Check sheet for the drawn part. Datum: minimum x, y, z corner. Units: mm. A direction names the side the tool comes from. Coordinates: 2 decimals unless noted, no trailing zeros. Loops run counter-clockwise (first coordinate to the right, second up) from the corner with the lowest first, then second, coordinate; pieces in that order, holes last. Notation, with made-up numbers: (32.5, -22.75) - (89.5, -22.75) arc R15 ccw to (89.5, -8.75) - close; hole circle Ø6 at (44.5, -25). An arc over 180 degrees is marked (long way). Answer as a JSON object with one key per item and string values. Group by question number.
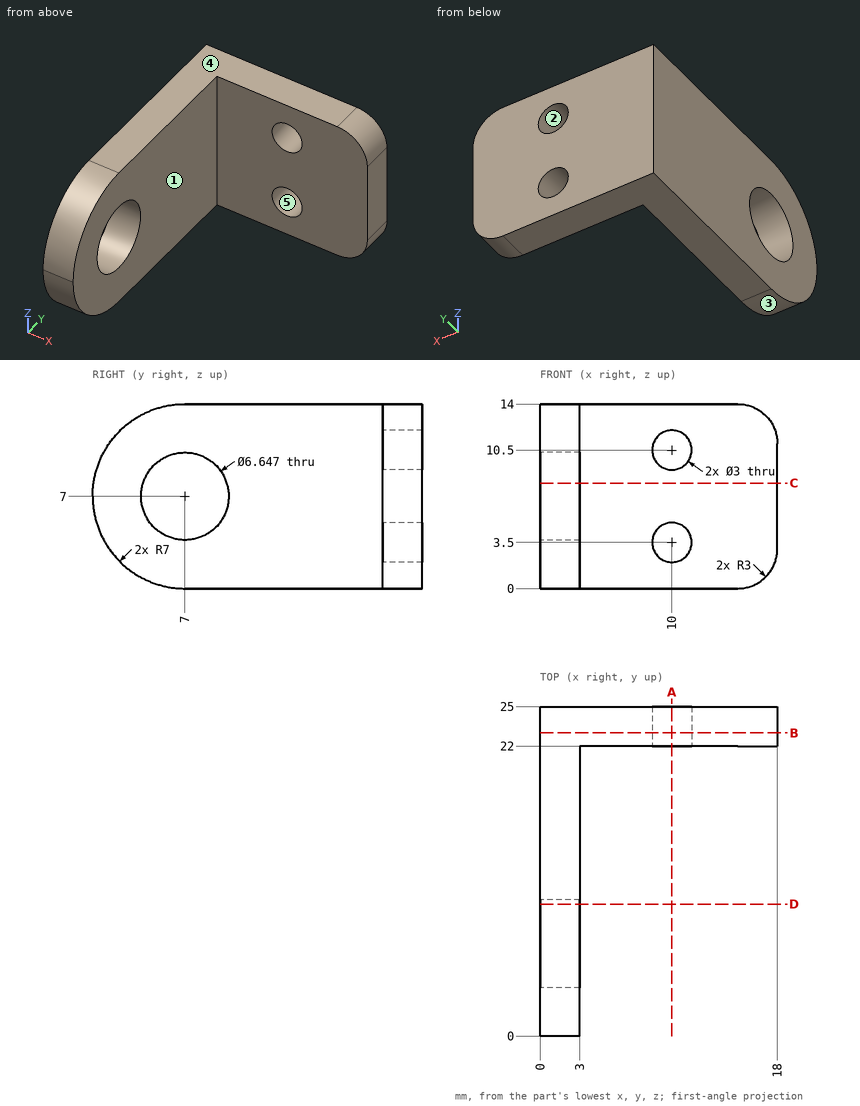
1. Sectioned sample at D-D on y = 10. Record the cut outline in (x, z).
2. Sectioned sample at A-A on x = 10. Record the cut outline in (y, z).
3. Access from +Z, -Z, +X, -X, +Y, -Y to the whole of each face (thin tool, end or side, straight path). Record for the marked faces 1 and 2.
4. Gauge pin test, flat ends, axial feed: pin 1 (1.5 mm diameter, centred on y = 9.5, z = 10.5, fed in from +X); pin 2 (4 mm diameter, centred on x = 14, z = 9.5, fed in from -Y); pin 3 (8 mm diameter, centred on x = 6, y = 10, fed in from -Z). Record the tip position at first contact, or that the pin passes through.
5. Release check for a two-part mould opening along Z. For the marked faces 3, 4 and 5 record: released by +Z, released by -Z, zero draft, split by the parting line, or undercut.
6. Sectioned sample at B-B on y = 23. Record the cut outline in (x, z), plus the area to 3 significant figures.
7. Sectioned sample at C-C on z = 8. Record the cut outline in (x, y).
8. Material ranges on line 1 (Z direction, x = 10, y = 24.05); line 2 (Z direction, x = 1.9, y = 7); line 3 (X direction, y = 23.85, z = 3.5), recorded low to high.
Answers follow:
{
 "1": {"outline": "(0, 0) - (3, 0) - (3, 5.57) - (0, 5.57) - close; (0, 8.43) - (3, 8.43) - (3, 14) - (0, 14) - close"},
 "2": {"outline": "(22, 0) - (25, 0) - (25, 2) - (22, 2) - close; (22, 5) - (25, 5) - (25, 9) - (22, 9) - close; (22, 12) - (25, 12) - (25, 14) - (22, 14) - close"},
 "3": {"face 1": "+Z, -Z, +X, -Y", "face 2": "+Y, -Y"},
 "4": {"pin 1": "stops at x = 3", "pin 2": "stops at y = 22", "pin 3": "stops at z = 0"},
 "5": {"face 3": "released by -Z", "face 4": "released by +Z", "face 5": "undercut"},
 "6": {"outline": "(0, 0) - (15, 0) arc R3 ccw to (18, 3) - (18, 11) arc R3 ccw to (15, 14) - (0, 14) - close; hole circle Ø3 at (10, 3.5); hole circle Ø3 at (10, 10.5)", "area": "234 mm^2"},
 "7": {"outline": "(0, 0.07) - (3, 0.07) - (3, 3.83) - (0, 3.83) - close; (0, 10.17) - (3, 10.17) - (3, 22) - (18, 22) - (18, 25) - (0, 25) - close"},
 "8": {"line 1": "z = 0 to 2, 5 to 9, 12 to 14", "line 2": "z = 0 to 3.68, 10.32 to 14", "line 3": "x = 0 to 8.5, 11.5 to 18"}
}
